Input: dimensioned drawing with shaded views. Units: mm. Origin: part minimum x, y, z. A direction names the side the tool comes from. Round coordinates to 2 decimals unless told otherwise and drop trailing zeros. Write each loop counter-clockwise with the first axis right and the second up, starting at its lowest first coordinate (ties: lowest second). Pieces come first, ordered by that corner, then holes. Notation, with made-up numbers: (-21, 63) - (-13, 63) arc R20 ccw to (-13, 69) - close; hole circle Ø4 at (29, -21.75). An arc over 180 degrees is marked (long way). Use one line per item in the form item = value.
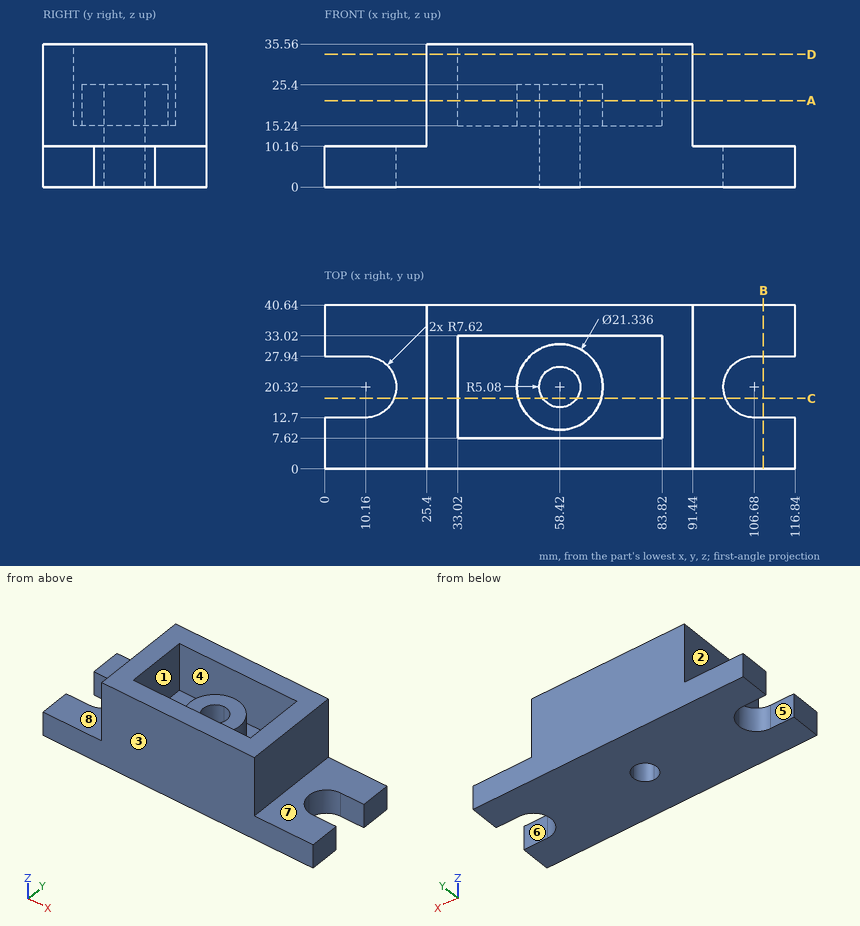
(1) Cut plane D-D on z = 33. Output: boundary loops of the cut face in (x, y), then the cut area to 3 significant figures.
Derived:
outline = (25.4, 0) - (91.44, 0) - (91.44, 40.64) - (25.4, 40.64) - close; hole (33.02, 7.62) - (83.82, 7.62) - (83.82, 33.02) - (33.02, 33.02) - close
area = 1,390 mm^2
(2) Cut plane C-C on y = 17.5. Output: boundary loops of the cut face in (x, z), then the cut area to 3 significant figures.
Derived:
outline = (17.24, 0) - (54.19, 0) - (54.19, 25.4) - (48.13, 25.4) - (48.13, 15.24) - (33.02, 15.24) - (33.02, 35.56) - (25.4, 35.56) - (25.4, 10.16) - (17.24, 10.16) - close; (62.65, 0) - (99.6, 0) - (99.6, 10.16) - (91.44, 10.16) - (91.44, 35.56) - (83.82, 35.56) - (83.82, 15.24) - (68.71, 15.24) - (68.71, 25.4) - (62.65, 25.4) - close
area = 1,480 mm^2
(3) Material intervals for L1, parallel to Y at x = 82, z = 34; L2, parallel to X at y = 20, z = 10; L3, parallel to X at y = 23, z = 21.5, sorted ascending.
Derived:
L1 = 0 to 7.62, 33.02 to 40.64
L2 = 17.77 to 53.35, 63.49 to 99.07
L3 = 25.4 to 33.02, 48.09 to 54.1, 62.74 to 68.75, 83.82 to 91.44
(4) Access query for the marked faces 4, 5, 6, 7 and 8. Directions: +Z, -Z, +X, -X, +Y, -Y. A direction counts if a zero-diameter tool reaches every point of the face in a straight line with its end or side. Return the directions, or none.
Derived:
face_4 = +Z
face_5 = +Z, -Z, -X
face_6 = +Z, -Z, +X
face_7 = +Z, +X, +Y, -Y
face_8 = +Z, -X, +Y, -Y
(5) Cut plane A-A on z = 21.5. Output: boundary loops of the cut face in (x, y).
Derived:
outline = (25.4, 0) - (91.44, 0) - (91.44, 40.64) - (25.4, 40.64) - close; circle Ø21.34 at (58.42, 20.32); hole (33.02, 7.62) - (83.82, 7.62) - (83.82, 33.02) - (33.02, 33.02) - close; hole circle Ø10.16 at (58.42, 20.32)
(6) Draft query along Y for the marked faces 1, 2 and 3. Return one class per face: released by +Y, released by -Y, zero draft, split by the parting line, or undercut.
Derived:
face_1 = undercut
face_2 = zero draft
face_3 = released by -Y
(7) Cut plane B-B on x = 109. Output: boundary loops of the cut face in (y, z).
Derived:
outline = (0, 0) - (12.7, 0) - (12.7, 10.16) - (0, 10.16) - close; (27.94, 0) - (40.64, 0) - (40.64, 10.16) - (27.94, 10.16) - close
(8) First-contact query: pin 1 Ø10 at (y, z) = (22, 29) entering from -X; pin 2 Ø12.5 at (x, y) = (105, 13) entering from +Z; pin 3 Ø7.5 at (y, z) = (17.5, 25) entering from +X; pin 4 Ø5 at (x, z) = (5.5, 4) entering from -Y. Flat tips, straight axial feed; report the tip coordinate or a pass-through.
Derived:
pin_1 = 25.4
pin_2 = 10.16
pin_3 = 91.44
pin_4 = 0
